```python
from build123d import *


# Read off the part's stored shape, not the designer's step: M8 Machine Threads Stud1
with BuildPart() as part:
    # Sketch1 → Revolve1 (revolve)
    with BuildSketch(Plane(origin=(0, 0, 0), x_dir=(1, 0, 0), z_dir=(0, 1, 0))):
        Polygon((0, 0), (0, 4), (1, 5), (2, 5), (2, 4), (3, 4), (3, 5), (26, 5), (26, 4.25), (41, 4.25), (41, 0), align=None)
    revolve(axis=Axis((41, 0, 0), (-1, 0, 0)))

    # M8 Machine Threads Stud1 outline → M8 Machine Threads Stud1 (revolve, cut)
    with BuildSketch(Plane.YX):
        Polygon((4.25, 41), (3.3095, 41), (4, 40.3095), (4, 26), (4.25, 26), align=None)
    revolve(axis=Axis((0, 0, 0), (1, 0, 0)), mode=Mode.SUBTRACT)


solid = part.part
```
Part model, mm, in its own coordinate system. A direction names the side the tool comes from. Round coordinates to 2 decimals unless told otherwise and drop trailing zeros. Loops run counter-clockwise (first coordinate to the right, second up) from the corner with the lowest first, then second, coordinate; pieces in that order, holes last.
1. 3-axis set-ups, long thin cutter, end or side, ignore diameter. For faces 1 (the face through (1.51, 4.88, 1.08)), 2 (the face through (33.055, -0.867, -3.905)): which of +Z, -Z, +X, -X, +Y, -Y reach the whole face in a straight line?
Solutions:
face 1: +X, -X
face 2: +X
2. Flat gauge pin, fed straight in: pin 1 (1.5 mm diameter, centred on x = 11, z = 2, fed in from +Y). Where does the tip first touch, or does it go through?
Solutions:
pin 1: stops at y = 4.84
3. Slice it at D-D (x = 32.5). Give the cut face in (y, z), and give its area (3 significant figures).
Solutions:
outline: circle Ø8 at (0, 0)
area: 50.3 mm2
4. Slice it at C-C (x = 15). Give the cut face in (y, z), and give its area (3 significant figures).
Solutions:
outline: circle Ø10 at (0, 0)
area: 78.5 mm2
5. Drill centre lines: line 1 along Z through (x, y) = (28, -0.25); line 2 along Y through (x, z) = (23.5, 3); line 3 along Y through (x, z) = (5.5, 3.75). Where is each one in solid material? Low to high.
Solutions:
line 1: z = -3.99 to 3.99
line 2: y = -4 to 4
line 3: y = -3.31 to 3.31
6. Slice it at A-A (z = 0). Give the cut face in (x, y), and give its area (3 significant figures).
Solutions:
outline: (0, -4) - (1, -5) - (2, -5) - (2, -4) - (3, -4) - (3, -5) - (26, -5) - (26, -4) - (40.31, -4) - (41, -3.31) - (41, 3.31) - (40.31, 4) - (26, 4) - (26, 5) - (3, 5) - (3, 4) - (2, 4) - (2, 5) - (1, 5) - (0, 4) - close
area: 377 mm2
7. Two-plate mould, pull along X, no slides. Class faces 3 (the face through (2.507, 3.905, 0.867)), 4 (the face through (14.66, 4.88, 1.08)), 5 (the face through (41, 0, 0)): pulls with the +X half, pulls with the -X half, needs draft (parallel to the pull), parting line crosses it, or undercut.
Solutions:
face 3: undercut
face 4: needs draft
face 5: pulls with the +X half
